```python
from build123d import *

# Parameters (mm, degrees)
F1_DEPTH       = 3
F2_D           = 4.3
F2_CBORE_D     = 7.5
F2_CBORE_DEPTH = 2
F3_D           = 4.3
F3_CBORE_D     = 7.5
F3_CBORE_DEPTH = 2
F4_R           = 5


with BuildPart() as f1:
    # F0 (on Front) → F1 (new body)
    with BuildSketch(Plane.XZ):
        with BuildLine():
            Line((10, 250), (-10, 250))
            Line((-10, 250), (-10, -250))
            Line((-10, -250), (10, -250))
            Line((10, -250), (10, -210))
            ThreePointArc((10, -210), (0, -200), (10, -190))
            Line((10, -190), (10, -10))
            ThreePointArc((10, -10), (0, 0), (10, 10))
            Line((10, 10), (10, 190))
            ThreePointArc((10, 190), (0, 200), (10, 210))
            Line((10, 210), (10, 250))
        make_face()
        with BuildLine():
            ThreePointArc((20, 200), (17.0710678119, 207.0710678119), (10, 210))
            Line((10, 210), (10, 190))
            ThreePointArc((10, 190), (17.0710678119, 192.9289321881), (20, 200))
        make_face()
        with BuildLine():
            Line((10, 190), (10, 210))
            ThreePointArc((10, 210), (0, 200), (10, 190))
        make_face()
        with BuildLine():
            ThreePointArc((10, -190), (0, -200), (10, -210))
            Line((10, -210), (10, -190))
        make_face()
        with BuildLine():
            Line((10, -190), (10, -210))
            ThreePointArc((10, -210), (17.0710678119, -207.0710678119), (20, -200))
            ThreePointArc((20, -200), (17.0710678119, -192.9289321881), (10, -190))
        make_face()
        with BuildLine():
            ThreePointArc((20, 0), (17.0710678119, 7.0710678119), (10, 10))
            Line((10, 10), (10, -10))
            ThreePointArc((10, -10), (17.0710678119, -7.0710678119), (20, 0))
        make_face()
        with BuildLine():
            Line((10, -10), (10, 10))
            ThreePointArc((10, 10), (0, 0), (10, -10))
        make_face()
    extrude(amount=F1_DEPTH)

    # F2 (through all)
    with Locations(Plane(origin=(0, 0, 0), x_dir=(1, 0, 0), z_dir=(0, 1, 0))):
        with Locations((0, 0), (0, -225), (0, 225)):
            CounterBoreHole(F2_D / 2, F2_CBORE_D / 2, F2_CBORE_DEPTH)

    # F3 (through all)
    with Locations(Plane(origin=(0, 0, 0), x_dir=(1, 0, 0), z_dir=(0, 1, 0))):
        with Locations((10, 0), (10, -200), (10, 200)):
            CounterBoreHole(F3_D / 2, F3_CBORE_D / 2, F3_CBORE_DEPTH)

    # F4
    f4_edges = [f1.edges().sort_by_distance(p)[0] for p in [
        (-10, -1.5, 250),
        (10, -1.5, 250),
        (-10, -1.5, -250),
        (10, -1.5, -250),
    ]]
    fillet(f4_edges, radius=F4_R)


solid = f1.part
```
Build history of the part. All positions in model axes, mm. Round coordinates to 2 decimals unless told otherwise and drop trailing zeros. Order: outer loops, then holes, each group sorted by start corner. A loop starts at its lowest first (then second) coordinate and runs counter-clockwise, first axis right, second up. Notation, with made-up numbers: (-20, -6) -> (11, -6) arc R27 cw to (11, 22) -> close; hole circle Ø3 at (35, 71). An arc over 180 degrees is marked (long way). Answer in a Markdown table with one row per item.
1) Band-saw the part on A-A on y = -1. Give the cut face in (x, z).
Values:
| item | result |
|---|---|
| outline | (-10, -245) arc R5 ccw to (-5, -250) -> (5, -250) arc R5 ccw to (10, -245) -> (10, -210) arc R10 ccw to (10, -190) -> (10, -10) arc R10 ccw to (10, 10) -> (10, 190) arc R10 ccw to (10, 210) -> (10, 245) arc R5 ccw to (5, 250) -> (-5, 250) arc R5 ccw to (-10, 245) -> close; hole circle Ø7.5 at (0, -225); hole circle Ø7.5 at (0, 0); hole circle Ø7.5 at (0, 225); hole circle Ø7.5 at (10, -200); hole circle Ø7.5 at (10, 0); hole circle Ø7.5 at (10, 200) |
2) Pin check, flat tips, straight feed: P1, Ø1, axis at y = -1, z = 74, coming from the +X side; P2, Ø7, axis at x = 0, z = 225, coming from the +Y side. Stop position of each tip, or through.
Values:
| item | result |
|---|---|
| P1 | x = 10 |
| P2 | y = -2 |
3) Wall check: L1, parallel to Z at x = 0, y = -2.25; L2, parallel to X at y = -2.7, z = 225; L3, parallel to Z at x = -2, y = -1.9. Give the ranges that are in metal, low to high.
Values:
| item | result |
|---|---|
| L1 | -250 to -227.15, -222.85 to -2.15, 2.15 to 222.85, 227.15 to 250 |
| L2 | -10 to -2.15, 2.15 to 10 |
| L3 | -250 to -228.17, -221.83 to -3.17, 3.17 to 221.83, 228.17 to 250 |
